from build123d import *

# Parameters (mm, degrees)
F0_R     = 3.5
F0_R_2   = 2
F1_DEPTH = 8
F2_R     = 2.3
F2_R_2   = 2
F3_DEPTH = 6
F4_R     = 3.5
F5_DEPTH = 2


with BuildPart() as f1:
    # F0 (on Top) → F1 (new body)
    with BuildSketch(Plane.XY):
        Circle(F0_R)
        Circle(F0_R_2, mode=Mode.SUBTRACT)
    extrude(amount=F1_DEPTH)

    # F2 (on face) → F3 (cut)
    with BuildSketch(Plane.XY.offset(8)):
        Circle(F2_R)
        Circle(F2_R_2, mode=Mode.SUBTRACT)
    extrude(amount=-F3_DEPTH, mode=Mode.SUBTRACT)

    # F4 (on Top) → F5 (join)
    with BuildSketch(Plane.XY):
        with BuildLine():
            Line((5.5, 4), (-5.5, 4))
            ThreePointArc((-5.5, 4), (-6.914214, 3.414214), (-7.5, 2))
            Line((-7.5, 2), (-7.5, -2))
            ThreePointArc((-7.5, -2), (-6.914214, -3.414214), (-5.5, -4))
            Line((-5.5, -4), (5.5, -4))
            ThreePointArc((5.5, -4), (6.914214, -3.414214), (7.5, -2))
            Line((7.5, -2), (7.5, 2))
            ThreePointArc((7.5, 2), (6.914214, 3.414214), (5.5, 4))
        make_face()
        Circle(F4_R, mode=Mode.SUBTRACT)
    extrude(amount=F5_DEPTH)


solid = f1.part
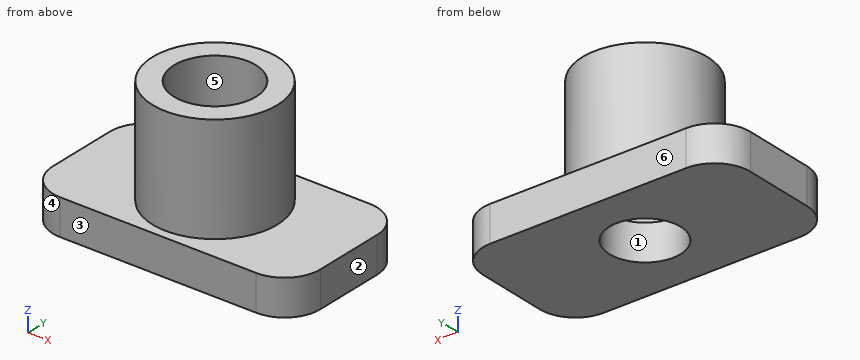
Input: part model. Units: mm. Frame: model coordinates. Face numbers are marked on the shaded views. A direction names the side the tool comes from. Coordinates: 2 decimals unless noted, no trailing zeros. Loops run counter-clockwise (first coordinate to the right, second up) from the corner with the lowest first, then second, coordinate; pieces in that order, holes last.
(1) Section B-B on z = 1.25. Return the cut outline in (x, y), then the cut area to 3 significant figures.
(2) Section A-A on y = 0. Return the cut outline in (x, z).
(3) Set-up query: the marked faces 5 and 6. Return all of +Z, -Z, +X, -X, +Y, -Y with unobstructed straight access to the full face (end or side cutting, diameter ignored); none if empty.
(4) Pull-direction query (X, two-part tool) for the marked faces 1, 2, 3 and 4; classes: released by +X, released by -X, zero draft, split by the parting line, or undercut.
(5) Section D-D on x = -5.25. Return the cut outline in (y, z), then the cut area to 3 significant figures.
(6) First-contact query: pin 1 Ø2.5 at (x, y) = (0, 0.5) entering from +Z; pin 2 Ø2 at (x, z) = (-3, 6) entering from +Y; pin 3 Ø1 at (x, z) = (0, 5) entering from -Y. Flat tips, straight axial feed; report the tip coordinate or a pass-through.
(7) Material intervals for probe 1 along Y at (x, z) = (0, 5.8); probe 2 along Z at (x, y) = (-4.25, 0.5); probe 3 along X at (y, z) = (0.25, 6.5), sorted ascending.
(8) Section C-C on x = 0. Return the cut outline in (y, z), then the cut area to 3 significant figures.
Data:
1. outline: (-7.5, -2) arc R2 ccw to (-5.5, -4) - (5.5, -4) arc R2 ccw to (7.5, -2) - (7.5, 2) arc R2 ccw to (5.5, 4) - (-5.5, 4) arc R2 ccw to (-7.5, 2) - close; hole circle Ø4 at (0, 0)
1. area: 104 mm2
2. outline: (-7.5, 0) - (-2, 0) - (-2, 2) - (-2.3, 2) - (-2.3, 8) - (-3.5, 8) - (-3.5, 2) - (-7.5, 2) - close; (2, 0) - (7.5, 0) - (7.5, 2) - (3.5, 2) - (3.5, 8) - (2.3, 8) - (2.3, 2) - (2, 2) - close
3. face 5: +Z
3. face 6: +Z, -Z, +X, -X, +Y
4. face 1: undercut
4. face 2: released by +X
4. face 3: zero draft
4. face 4: released by -X
5. outline: (-4, 0) - (4, 0) - (4, 2) - (-4, 2) - close
5. area: 16.0 mm2
6. pin 1: passes through
6. pin 2: stops at y = 2.87
6. pin 3: stops at y = -3.5
7. probe 1: y = -3.5 to -2.3, 2.3 to 3.5
7. probe 2: z = 0 to 2
7. probe 3: x = -3.49 to -2.29, 2.29 to 3.49
8. outline: (-4, 0) - (-2, 0) - (-2, 2) - (-2.3, 2) - (-2.3, 8) - (-3.5, 8) - (-3.5, 2) - (-4, 2) - close; (2, 0) - (4, 0) - (4, 2) - (3.5, 2) - (3.5, 8) - (2.3, 8) - (2.3, 2) - (2, 2) - close
8. area: 22.4 mm2
